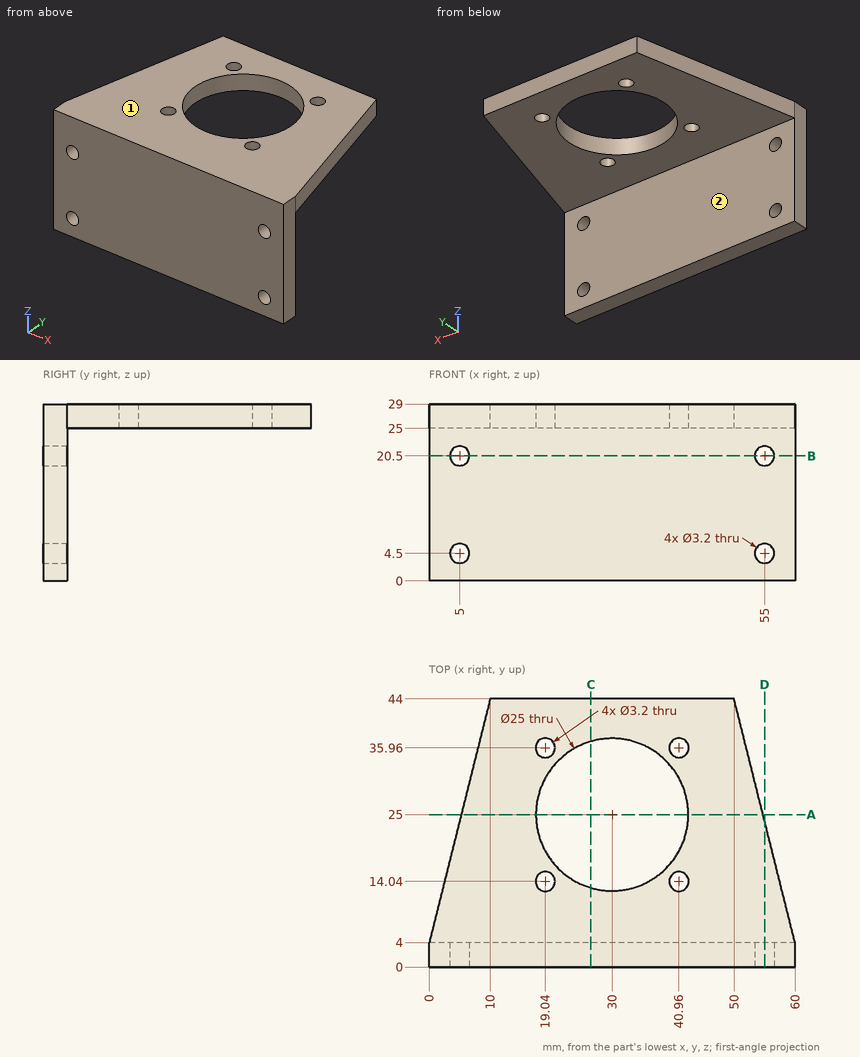
The drawing under review shows one solid part. Ordinate dimensions are in mm from its lowest x, y, z. A direction names the side the tool comes from. Round coordinates to 2 decimals unless told otherwise and drop trailing zeros. Order: outer loops, then holes, each group sorted by start corner. A loop starts at its lowest first (then second) coordinate and runs counter-clockwise, first axis right, second up. Notation, with made-up numbers: (-5.75, 87) - (28.25, 87) arc R37 cw to (28.25, 125) - close; hole circle Ø4 at (30, 44). An arc over 180 degrees is marked (long way). Return JSON: item names as keys, results as strings.
Q1. Consider section D-D on x = 55. Write out the cut boundary in (y, z), plus the area to 3 significant figures.
Computed values:
{"outline": "(0, 0) - (4, 0) - (4, 2.9) - (0, 2.9) - close; (0, 6.1) - (4, 6.1) - (4, 18.9) - (0, 18.9) - close; (0, 22.1) - (4, 22.1) - (4, 25) - (24, 25) - (24, 29) - (0, 29) - close", "area": "170 mm2"}
Q2. Consider section B-B on z = 20.5. Write out the cut boundary in (x, y), plus the area to 3 significant figures.
Computed values:
{"outline": "(0, 0) - (3.4, 0) - (3.4, 4) - (0, 4) - close; (6.6, 0) - (53.4, 0) - (53.4, 4) - (6.6, 4) - close; (56.6, 0) - (60, 0) - (60, 4) - (56.6, 4) - close", "area": "214 mm2"}
Q3. Consider section C-C on x = 26.5. Write out the cut boundary in (y, z), plus the area to 3 significant figures.
Computed values:
{"outline": "(0, 0) - (4, 0) - (4, 25) - (13, 25) - (13, 29) - (0, 29) - close; (37, 25) - (44, 25) - (44, 29) - (37, 29) - close", "area": "180 mm2"}
Q4. Machinability: for the marked faces 1 and 2, which of the approach directions +Z, -Z, +X, -X, +Y, -Y give a long, thin tool a straight path to every point of the face, cutting with its end or side? Answer none if there is none.
Computed values:
{"face 1": "+Z, +X, -X, +Y, -Y", "face 2": "-Z, +X, -X, +Y"}
Q5. Consider section A-A on y = 25. Write out the cut boundary in (x, z), plus the area to 3 significant figures.
Computed values:
{"outline": "(5.25, 25) - (17.5, 25) - (17.5, 29) - (5.25, 29) - close; (42.5, 25) - (54.75, 25) - (54.75, 29) - (42.5, 29) - close", "area": "98.0 mm2"}
Q6. Wall thickness on L1, parallel to X at y = 2.05, z = 4.5; L2, parallel to Y at x = 27.5, z = 15.5; L3, parallel to Y at x = 30, z = 27.5: over which ranges is each line inside the solid? List them lowest first. Write a range as [from, to].
Computed values:
{"L1": "x = [0, 3.4], [6.6, 53.4], [56.6, 60]", "L2": "y = [0, 4]", "L3": "y = [0, 12.5], [37.5, 44]"}
Q7. For pin 1 Ø1.9 at (x, z) = (55, 4.5) entering from +Y; pin 2 Ø6 at (x, z) = (34, 14.5) entering from +Y; pin 3 Ø5 at (x, y) = (19.04, 35.96) entering from -Z, all flat-tipped, find the tip position at first contact; note any pin that passes through.
Computed values:
{"pin 1": "passes through", "pin 2": "stops at y = 4", "pin 3": "stops at z = 25"}
